Work out the finished part from the listing and answer in its coordinate system (mm). A direction names the side the tool comes from. Coordinates: 2 decimals unless noted, no trailing zeros. Order: outer loops, then holes, each group sorted by start corner. A loop starts at its lowest first (then second) coordinate and runs counter-clockwise, first axis right, second up. Notation, with made-up numbers: (8, -32) -> (26, -32) arc R16 cw to (26, -27) -> close; hole circle Ø6 at (-34, 24). An arc over 180 degrees is marked (long way). Use one line per item in the form item = value.
from build123d import *

# Parameters (mm, degrees)
F1_DEPTH = 200
F3_DEPTH = 150
F4_R     = 100
F5_DEPTH = 350.001


with BuildPart() as f1:
    # F0 (on Front) → F1 (new body)
    with BuildSketch(Plane.XZ):
        with BuildLine():
            Line((-300, 300), (-300, -300))
            Line((-300, -300), (-180, -300))
            ThreePointArc((-180, -300), (0, -120), (180, -300))
            Line((180, -300), (300, -300))
            Line((300, -300), (300, 300))
            ThreePointArc((300, 300), (0, 600), (-300, 300))
        make_face()
    extrude(amount=F1_DEPTH)

    # F2 (on face) → F3 (join)
    with BuildSketch(Plane.XZ.offset(200)):
        with BuildLine():
            Line((-179.99268, 540.00549), (-179.934111, 59.950597))
            ThreePointArc((-179.934111, 59.950597), (0.082353, 1.1e-05), (180.065876, 60.049421))
            Line((180.065876, 60.049421), (180.00732, 539.99451))
            ThreePointArc((180.00732, 539.99451), (0.00915, 600), (-179.99268, 540.00549))
        make_face()
    extrude(amount=F3_DEPTH)

    # F4 (on face) → F5 (cut, through all)
    with BuildSketch(Plane.XZ.offset(350)):
        with Locations((0, 300)):
            Circle(F4_R)
    extrude(amount=-F5_DEPTH, mode=Mode.SUBTRACT)


solid = f1.part
(1) Which of the six approach directions +Z, -Z, +X, -X, +Y, -Y give full straight-line access (tool end or side, diameter ignored) to faces 1 (the flat face through (-82, -350, 371)), 2 (the flat face through (-4, -200, -61))?
Data:
face_1 = +Z, -Z, +X, -X, -Y
face_2 = -Z, -Y
(2) Section C-C on z = -133 is taken. Write down the section's boundary in (x, y), plus the area to 3 significant figures.
Data:
outline = (-300, -200) -> (-67.16, -200) -> (-67.16, 0) -> (-300, 0) -> close; (67.16, -200) -> (300, -200) -> (300, 0) -> (67.16, 0) -> close
area = 93,100 mm²
(3) Straight lines are drawn through the part: line 1 along X through (y, z) = (-276.5, 403.5); line 2 along Z through (x, y) = (0, -253); line 3 along Y through (x, z) = (-99.5, -141). For each, find the intervals that lie inside material, in ascending order.
Data:
line_1 = -179.98 to 180.02
line_2 = 0 to 200, 400 to 600
line_3 = -200 to 0
(4) Section D-D on x = 86 is taken. Write down the section's boundary in (y, z).
Data:
outline = (-350, 12.59) -> (-200, 12.59) -> (-200, -141.87) -> (0, -141.87) -> (0, 248.97) -> (-350, 248.97) -> close; (-350, 351.03) -> (0, 351.03) -> (0, 587.41) -> (-350, 587.41) -> close
(5) Section B-B on y = -34.5 is taken. Write down the section's boundary in (x, z).
Data:
outline = (-300, -300) -> (-180, -300) arc R180 cw to (180, -300) -> (300, -300) -> (300, 300) arc R300 ccw to (-300, 300) -> close; hole circle Ø200 at (0, 300)
(6) Section A-A on x = 0 is taken. Write down the section's boundary in (y, z), plus the area to 3 significant figures.
Data:
outline = (-350, 0) -> (-200, 0) -> (-200, -120) -> (0, -120) -> (0, 200) -> (-350, 200) -> close; (-350, 400) -> (0, 400) -> (0, 600) -> (-350, 600) -> close
area = 164,000 mm²
(7) Each of these flat-tipped pins is pushed along its axis until it touches: P1, Ø12, axis at y = -292.5, z = 176.5, coming from the +X side; P2, Ø12, axis at y = -264, z = 414, coming from the -X side; P3, Ø12, axis at x = -58.5, y = -77, coming from the +Z side. Where does it stop, or does it pass through?
Data:
P1 = 180.05
P2 = -179.98
P3 = 595.37
